Design review of the part built by this model. Coordinates are the model's own, in mm. A direction names the side the tool comes from. Coordinates: 2 decimals unless noted, no trailing zeros. Loops run counter-clockwise (first coordinate to the right, second up) from the corner with the lowest first, then second, coordinate; pieces in that order, holes last. Notation, with made-up numbers: (22, -24.75) -> (51, -24.75) arc R16 ccw to (51, -11.75) -> close; hole circle Ø3 at (5.5, 68.5). An arc over 180 degrees is marked (long way). Answer in a Markdown table with one row per item.
```python
from build123d import *

# Parameters (mm, degrees)
F0_W     = 38.1
F0_H     = 76.2
F1_DEPTH = 25.4
F3_DEPTH = 22.86
F4_D     = 2.2606
F4_DEPTH = 14.605
F4_TIP   = 0.6791527577
F5_R     = 2.54


with BuildPart() as f1:
    # F0 (on Top) → F1 (new body)
    with BuildSketch(Plane.XY):
        Rectangle(F0_W, F0_H)
    extrude(amount=F1_DEPTH)

    # F2 (on Top) → F3 (cut)
    with BuildSketch(Plane.XY):
        Polygon((10.16, 36.1509363616), (-10.16, 36.1509363616), (-10.16, 29.8009363616), (-16.51, 29.8009363616), (-16.51, -28.6190636384), (-10.16, -28.6190636384), (-10.16, -34.9690636384), (10.16, -34.9690636384), (10.16, -28.6190636384), (16.51, -28.6190636384), (16.51, 29.8009363616), (10.16, 29.8009363616), align=None)
    extrude(amount=F3_DEPTH, mode=Mode.SUBTRACT)

    # F4
    with Locations(Plane(origin=(0, 0, 0), x_dir=(1, 0, 0), z_dir=(0, 0, -1))):
        with Locations((-14.605, -33.655), (14.605, -33.655), (14.605, 33.655), (-14.605, 33.0640636384)):
            Hole(F4_D / 2, depth=F4_DEPTH)
            with Locations((0, 0, -(F4_DEPTH + F4_TIP / 2))):  # 118° drill point
                Cone(0, F4_D / 2, F4_TIP, mode=Mode.SUBTRACT)

    # F5
    f5_edges = [f1.edges().sort_by_distance(p)[0] for p in [
        (19.05, -38.1, 12.7),
        (-19.05, -38.1, 12.7),
        (-19.05, 38.1, 12.7),
        (19.05, 38.1, 12.7),
    ]]
    fillet(f5_edges, radius=F5_R)


solid = f1.part
```
(1) Tool access review of faces 5 (the cylindrical face through (18.286, 37.376, 12.878)), 6 (the flat face through (0, 36.151, 11)): name each direction out of +Z, -Z, +X, -X, +Y, -Y from which nothing blocks a thin tool from reaching the whole face with its end or side.
Evaluation:
| item | result |
|---|---|
| face 5 | +Z, -Z, +X, +Y |
| face 6 | -Z |
(2) Take a section at C-C on y = -19. Give the boundary of the cut face in (x, z).
Evaluation:
| item | result |
|---|---|
| outline | (-19.05, 0) -> (-16.51, 0) -> (-16.51, 22.86) -> (16.51, 22.86) -> (16.51, 0) -> (19.05, 0) -> (19.05, 25.4) -> (-19.05, 25.4) -> close |
(3) For pin 1 (10 mm diameter, centred on x = 3.5, y = -17, fed in from -Z), flat-tipped, find the tip position at first contact; note if it passes through.
Evaluation:
| item | result |
|---|---|
| pin 1 | stops at z = 22.86 |
(4) Take a section at D-D on z = 3.5. Give the boundary of the cut face in (x, y) (3 decimals), and give its area (3 significant figures).
Evaluation:
| item | result |
|---|---|
| outline | (-19.05, -35.56) arc R2.54 ccw to (-16.51, -38.1) -> (16.51, -38.1) arc R2.54 ccw to (19.05, -35.56) -> (19.05, 35.56) arc R2.54 ccw to (16.51, 38.1) -> (-16.51, 38.1) arc R2.54 ccw to (-19.05, 35.56) -> close; hole (-16.51, -28.619) -> (-10.16, -28.619) -> (-10.16, -34.969) -> (10.16, -34.969) -> (10.16, -28.619) -> (16.51, -28.619) -> (16.51, 29.801) -> (10.16, 29.801) -> (10.16, 36.151) -> (-10.16, 36.151) -> (-10.16, 29.801) -> (-16.51, 29.801) -> close; hole circle Ø2.261 at (-14.605, -33.064); hole circle Ø2.261 at (-14.605, 33.655); hole circle Ø2.261 at (14.605, -33.655); hole circle Ø2.261 at (14.605, 33.655) |
| area | 695 mm² |
(5) Take a section at B-B on x = 6. Give the boundary of the cut face in (y, z), and give its area (3 significant figures).
Evaluation:
| item | result |
|---|---|
| outline | (-38.1, 0) -> (-34.97, 0) -> (-34.97, 22.86) -> (36.15, 22.86) -> (36.15, 0) -> (38.1, 0) -> (38.1, 25.4) -> (-38.1, 25.4) -> close |
| area | 310 mm² |
(6) To check wall thickness, follow probe 1 along X at (y, z) = (-23, 14.75); probe 2 along X at (y, z) = (30.5, 11.75); probe 3 along Y at (x, z) = (9.5, 12.5). State the ranges of each line that lie inside material, in increasing order.
Evaluation:
| item | result |
|---|---|
| probe 1 | x = -19.05 to -16.51, 16.51 to 19.05 |
| probe 2 | x = -19.05 to -10.16, 10.16 to 19.05 |
| probe 3 | y = -38.1 to -34.97, 36.15 to 38.1 |
(7) Take a section at A-A on z = 21.25. Give the boundary of the cut face in (x, y), and give its area (3 significant figures).
Evaluation:
| item | result |
|---|---|
| outline | (-19.05, -35.56) arc R2.54 ccw to (-16.51, -38.1) -> (16.51, -38.1) arc R2.54 ccw to (19.05, -35.56) -> (19.05, 35.56) arc R2.54 ccw to (16.51, 38.1) -> (-16.51, 38.1) arc R2.54 ccw to (-19.05, 35.56) -> close; hole (-16.51, -28.62) -> (-10.16, -28.62) -> (-10.16, -34.97) -> (10.16, -34.97) -> (10.16, -28.62) -> (16.51, -28.62) -> (16.51, 29.8) -> (10.16, 29.8) -> (10.16, 36.15) -> (-10.16, 36.15) -> (-10.16, 29.8) -> (-16.51, 29.8) -> close |
| area | 711 mm² |
(8) Draft analysis for pull direction Y (two halves, no side actions). For faces 1 (the flat face through (0, -34.969, 11)), 2 (the cylindrical face through (-18.326, 37.336, 12.878)), 3 (the cylindrical face through (-18.326, -37.336, 12.878)), 4 (the conical face through (14.562, 33.847, 15.166)), state which applies: pulls with the +Y half, pulls with the -Y half, needs draft (parallel to the pull), parting line crosses it, or undercut.
Evaluation:
| item | result |
|---|---|
| face 1 | undercut |
| face 2 | pulls with the +Y half |
| face 3 | pulls with the -Y half |
| face 4 | undercut |
